Design review of the part shown in the three views and the two pictorial views. Dimensions are in mm from the part's minimum x, y and z. A direction names the side the tool comes from. Round coordinates to 2 decimals unless told otherwise and drop trailing zeros. Order: outer loops, then holes, each group sorted by start corner. A loop starts at its lowest first (then second) coordinate and runs counter-clockwise, first axis right, second up.
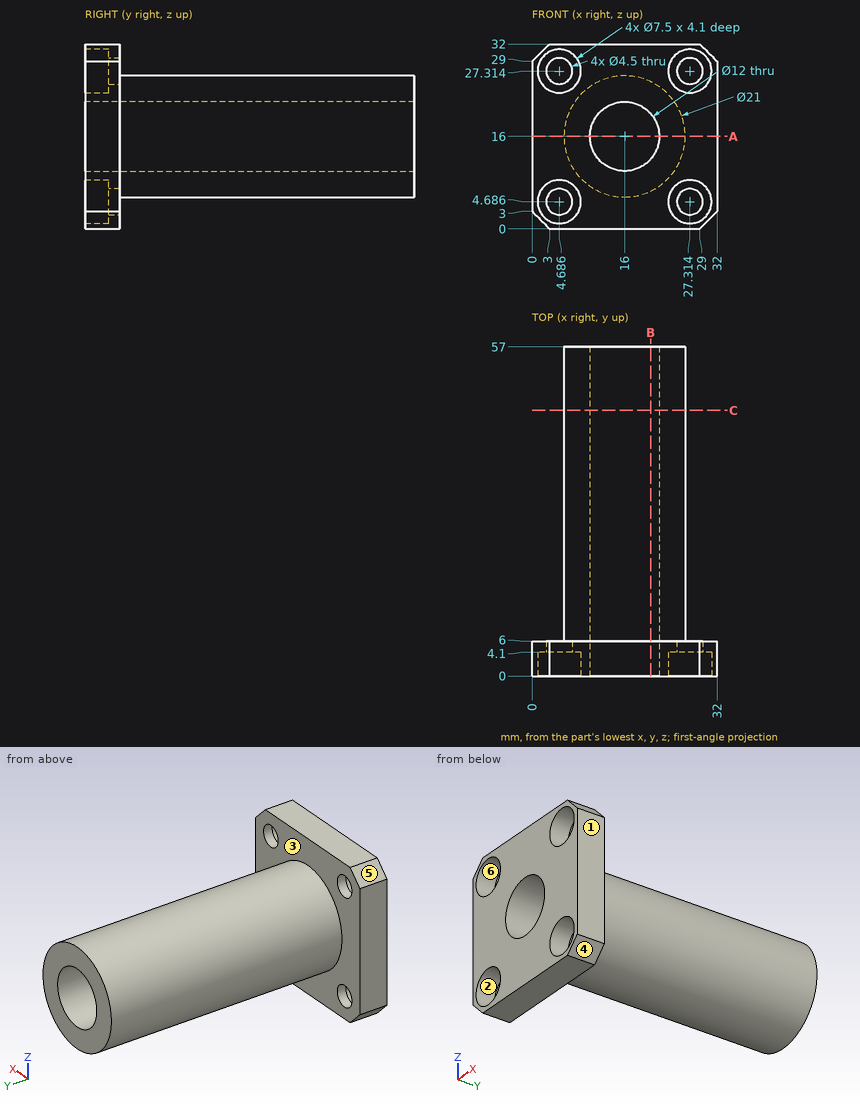
1) For the marked faces 1, 2 and 3, list the 3-axis set-ups (+Z, -Z, +X, -X, +Y, -Y) from which the entire face can be reached by the end or side of a thin tool; tool diameter is ignored.
Results:
face 1: +Z, -Z, +X, +Y, -Y
face 2: -Y
face 3: +Y
2) The part is to be moulded in two halves that separate along X. For the marked faces 4, 5 and 6, say which applies: released by +X, released by -X, zero draft, split by the parting line, or undercut.
Results:
face 4: released by +X
face 5: released by -X
face 6: undercut
3) Take a section at C-C on y = 46. Give the boundary of the cut face in (x, z).
Results:
outline: circle Ø21 at (16, 16); hole circle Ø12 at (16, 16)
4) To check wall thickness, follow line 1 along X through (y, z) = (35, 16); line 2 along X through (y, z) = (2.5, 21.5) (1 decimal); line 3 along Y through (x, z) = (11.5, 5). State the ranges of each line that lie inside material, in increasing order.
Results:
line 1: x = 5.5 to 10, 22 to 26.5
line 2: x = 0 to 13.6, 18.4 to 32
line 3: y = 0 to 6
5) Clearance check with flat-ended pins moving along their axes: P1, Ø1, axis at x = 4, y = 19, coming from the +Z side; P2, Ø1.5, axis at x = 8, y = 34.5, coming from the +Z side (1 decimal); P3, Ø5, axis at x = 27.31, z = 27.31, coming from the -Y side; P4, Ø1.5, axis at x = 22.5, y = 35, coming from the -Z side (1 decimal). State where each tip first meets the part, or that it passes through.
Results:
P1: passes through
P2: stops at z = 23.6
P3: stops at y = 4.1
P4: stops at z = 7.2
6) Take a section at A-A on z = 16. Give the boundary of the cut face in (x, y), plus the area to 3 significant figures.
Results:
outline: (0, 0) - (10, 0) - (10, 57) - (5.5, 57) - (5.5, 6) - (0, 6) - close; (22, 0) - (32, 0) - (32, 6) - (26.5, 6) - (26.5, 57) - (22, 57) - close
area: 579 mm2
7) Take a section at B-B on x = 20.5. Give the boundary of the cut face in (y, z), plus the area to 3 significant figures.
Results:
outline: (0, 0) - (6, 0) - (6, 6.51) - (57, 6.51) - (57, 12.03) - (0, 12.03) - close; (0, 19.97) - (57, 19.97) - (57, 25.49) - (6, 25.49) - (6, 32) - (0, 32) - close
area: 707 mm2
